```python
from build123d import *

# Parameters (mm, degrees)
SKETCH_R      = 56.5
PAD_DEPTH     = 2
FILLET_R      = 1.7
SKETCH001_R   = 45.75
SKETCH001_R_2 = 44.75
PAD001_DEPTH  = 23
POCKET_DEPTH  = 0.7
FILLET001_R   = 0.3


with BuildPart() as part:
    # Sketch → Pad (new body)
    with BuildSketch(Plane.XY):
        Circle(SKETCH_R)
    extrude(amount=PAD_DEPTH)

    # Fillet
    fillet_edges = [part.edges().sort_by_distance(p)[0] for p in [
        (-56.5, 0, 0),
    ]]
    fillet(fillet_edges, radius=FILLET_R)

    # Sketch001 (on Face3 of Fillet) → Pad001 (join)
    with BuildSketch(Plane.XY.offset(2)):
        Circle(SKETCH001_R)
        Circle(SKETCH001_R_2, mode=Mode.SUBTRACT)
    extrude(amount=PAD001_DEPTH)

    # Sketch002 (on Face3 of Pad001) → Pocket (cut)
    with BuildSketch(Plane.XY.offset(2)):
        with BuildLine():
            Line((-64, 7.5), (-49.8, 7.5))
            ThreePointArc((-47.8, 5.5), (-48.385786, 6.914214), (-49.8, 7.5))
            Line((-47.8, 5.5), (-47.8, -5.5))
            ThreePointArc((-49.8, -7.5), (-48.385786, -6.914214), (-47.8, -5.5))
            Line((-49.8, -7.5), (-64, -7.5))
            Line((-64, -7.5), (-64, 7.5))
        make_face()
        with BuildLine():
            Line((49.8, 7.5), (64.06, 7.5))
            Line((64.06, 7.5), (64.06, -7.5))
            Line((64.06, -7.5), (49.8, -7.5))
            ThreePointArc((47.8, -5.5), (48.385786, -6.914214), (49.8, -7.5))
            Line((47.8, -5.5), (47.8, 5.5))
            ThreePointArc((49.8, 7.5), (48.385786, 6.914214), (47.8, 5.5))
        make_face()
    extrude(amount=-POCKET_DEPTH, mode=Mode.SUBTRACT)

    # Fillet001
    fillet001_edges = [part.edges().sort_by_distance(p)[0] for p in [
        (52.875922, 7.5, 1.3),
        (48.385786, 6.914214, 1.3),
        (47.8, 0, 1.3),
        (48.385786, -6.914214, 1.3),
        (52.875922, -7.5, 1.3),
        (-52.875922, 7.5, 1.3),
        (-48.385786, 6.914214, 1.3),
        (-47.8, 0, 1.3),
        (-48.385786, -6.914214, 1.3),
        (-52.875922, -7.5, 1.3),
    ]]
    fillet(fillet001_edges, radius=FILLET001_R)


solid = part.part
```
Design review of the part built by this model. Coordinates are the model's own, in mm. A direction names the side the tool comes from. Coordinates: 2 decimals unless noted, no trailing zeros. Write each loop counter-clockwise with the first axis right and the second up, starting at its lowest first coordinate (ties: lowest second). Pieces come first, ordered by that corner, then holes. Notation, with made-up numbers: M 77,77 L 111,77 A18 cw 111,111 Z; hole C 71,17 d11. An arc over 180 degrees is marked long. Answer as a JSON object with one key per item and string values.
Item 1: Draft analysis for pull direction Y (two halves, no side actions). For faces 1 (the flat face through (-1, 1, 2)), 2 (the cylindrical face through (43.64, 13.74, 13.34)), 3 (the cylindrical face through (-1.14, -56.49, 1.85)), 4 (the flat face through (10, -44, 25)), state which applies: pulls with the +Y half, pulls with the -Y half, needs draft (parallel to the pull), parting line crosses it, or undercut.
Outcome:
{"face 1": "undercut", "face 2": "parting line crosses it", "face 3": "pulls with the -Y half", "face 4": "needs draft"}
Item 2: Add section C-C, the plane z = 11. Give the boundary of the cut face in (x, y), and give its area (3 significant figures).
Outcome:
{"outline": "C 0,0 d91.5; hole C 0,0 d89.5", "area": "284 mm²"}
Item 3: Wall thickness on probe 1 along Y at (x, z) = (0, 20.25); probe 2 along Z at (x, y) = (13, 16.5); probe 3 along X at (y, z) = (-35, 24.25): over which ranges is each line inside the solid? List them lowest first.
Outcome:
{"probe 1": "-45.75 to -44.75, 44.75 to 45.75", "probe 2": "0 to 2", "probe 3": "-29.46 to -27.88, 27.88 to 29.46"}
Item 4: Machinability: for faces 5 (the flat face through (52, 0, 1.3)), 6 (the flat face through (-1, 1, 0)), 7 (the flat face through (-46, 0, 2)), 8 (the flat face through (-52, 0, 1.3)), 9 (the cylindrical face through (1.14, 56.49, 1.85)), which of the approach directions +Z, -Z, +X, -X, +Y, -Y give a long, thin tool a straight path to every point of the face, cutting with its end or side? Answer none if there is none.
Outcome:
{"face 5": "+Z, +X", "face 6": "-Z, +X, -X, +Y, -Y", "face 7": "+Z", "face 8": "+Z, -X", "face 9": "+Z, -Z, +Y"}
Item 5: Insertion check: pin 1 Ø9 at (x, y) = (52.5, -3.5) entering from +Z; pin 2 Ø3 at (y, z) = (31.5, 7) entering from -X; pin 3 Ø9 at (x, y) = (-53.5, -1.5) entering from +Z; pin 4 Ø6 at (x, y) = (-21.5, 28) entering from -Z. Each pin has a flat end and moves straight along its axis. Give the tip position at first contact, or say it passes through.
Outcome:
{"pin 1": "z = 2", "pin 2": "x = -34.54", "pin 3": "z = 1.3", "pin 4": "z = 0"}
Item 6: Add section B-B, the plane y = 0. Give the boundary of the cut face in (x, z).
Outcome:
{"outline": "M -56.45,1.3 A1.7 ccw -54.8,0 L 54.8,0 A1.7 ccw 56.45,1.3 L 48.1,1.3 A0.3 cw 47.8,1.6 L 47.8,2 L 45.75,2 L 45.75,25 L 44.75,25 L 44.75,2 L -44.75,2 L -44.75,25 L -45.75,25 L -45.75,2 L -47.8,2 L -47.8,1.6 A0.3 cw -48.1,1.3 Z"}
Item 7: Add section A-A, the plane x = 0. Give the boundary of the cut face in (y, z).
Outcome:
{"outline": "M -56.5,1.7 A1.7 ccw -54.8,0 L 54.8,0 A1.7 ccw 56.5,1.7 L 56.5,2 L 45.75,2 L 45.75,25 L 44.75,25 L 44.75,2 L -44.75,2 L -44.75,25 L -45.75,25 L -45.75,2 L -56.5,2 Z"}
